Answer from the drawing. Dimensions are ordinates in mm from the lowest x, y and z of the part. A direction names the side the tool comes from. Coordinates: 2 decimals unless noted, no trailing zeros. Write each loop counter-clockwise with the first axis right and the second up, starting at its lowest first coordinate (ties: lowest second). Pieces come first, ordered by that corner, then holes.
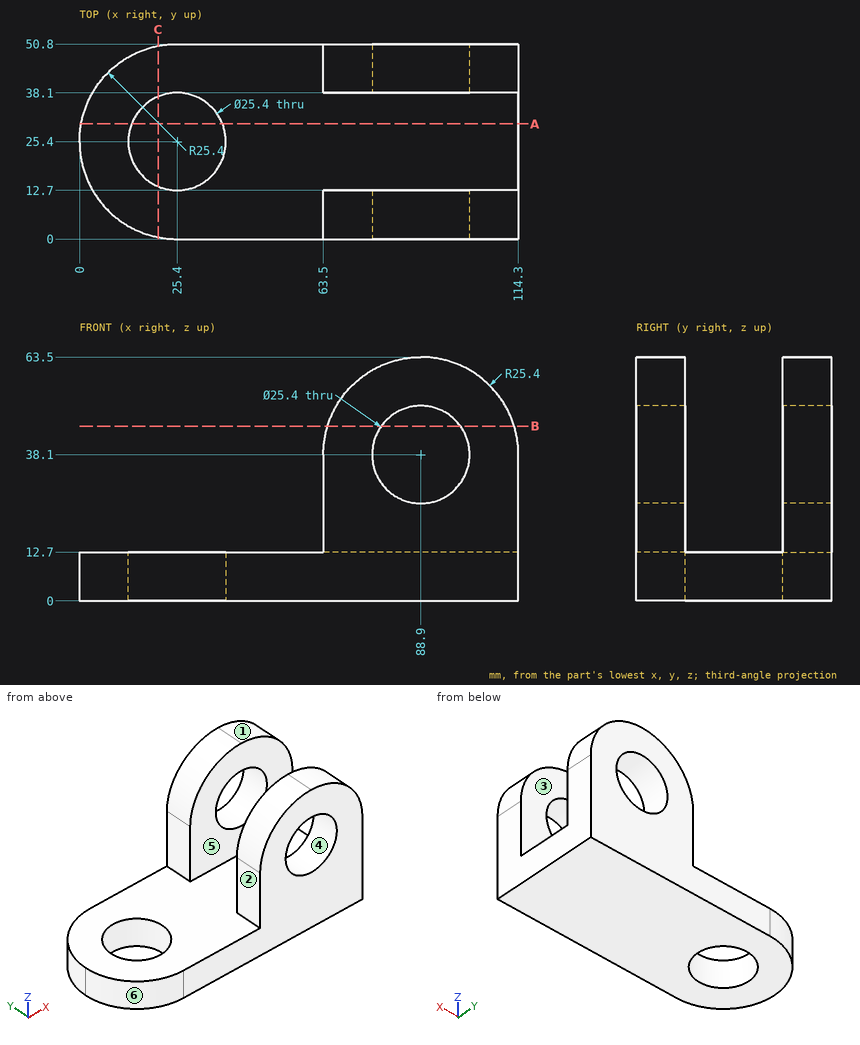
(1) Section A-A, the plane y = 30 is taken. Write down the section's boundary in (x, z), plus the area to 3 significant figures.
(2) Section B-B, the plane z = 45.5 is taken. Write down the section's boundary in (x, y), plus the area to 3 significant figures.
(3) For a pull along X with two mould halves and no side action, classify the marked faces 4, 5 and 6 as pulls with the +X half, pulls with the -X half, needs draft (parallel to the pull), parting line crosses it, or undercut.
(4) Each of these flat-tipped pins is pushed along its axis until it touches: pin 1 (14 mm diameter, centred on y = 7, z = 31, fed in from -X); pin 2 (15 mm diameter, centred on x = 88.9, z = 38.1, fed in from -Y); pin 3 (12 mm diameter, centred on x = 11.5, y = 10, fed in from +Z). Where does it stop, or does it pass through?
(5) Find the intervals of material crossed by probe 1 along Y at (x, z) = (75.5, 25); probe 2 along Z at (x, y) = (104, 28); probe 3 along X at (y, z) = (43, 38), in increasing order.
(6) Which of the six approach directions +Z, -Z, +X, -X, +Y, -Y give full straight-line access (tool end or side, diameter ignored) to the marked faces 1, 2 and 3?
(7) Section C-C, the plane x = 20.5 is taken. Write down the section's boundary in (y, z).
Solution:
1. outline: (0.42, 0) - (13.56, 0) - (13.56, 12.7) - (0.42, 12.7) - close; (37.24, 0) - (114.3, 0) - (114.3, 12.7) - (37.24, 12.7) - close
1. area: 1,150 mm2
2. outline: (64.6, 0) - (78.58, 0) - (78.58, 12.7) - (64.6, 12.7) - close; (64.6, 38.1) - (78.58, 38.1) - (78.58, 50.8) - (64.6, 50.8) - close; (99.22, 0) - (113.2, 0) - (113.2, 12.7) - (99.22, 12.7) - close; (99.22, 38.1) - (113.2, 38.1) - (113.2, 50.8) - (99.22, 50.8) - close
2. area: 710 mm2
3. face 4: undercut
3. face 5: needs draft
3. face 6: pulls with the -X half
4. pin 1: stops at x = 63.5
4. pin 2: passes through
4. pin 3: stops at z = 12.7
5. probe 1: y = 0 to 12.7, 38.1 to 50.8
5. probe 2: z = 0 to 12.7
5. probe 3: x = 63.5 to 76.2, 101.6 to 114.3
6. face 1: +Z, +X, +Y, -Y
6. face 2: +Z, -X, +Y, -Y
6. face 3: +Z, +X, -X
7. outline: (0.48, 0) - (13.68, 0) - (13.68, 12.7) - (0.48, 12.7) - close; (37.12, 0) - (50.32, 0) - (50.32, 12.7) - (37.12, 12.7) - close
